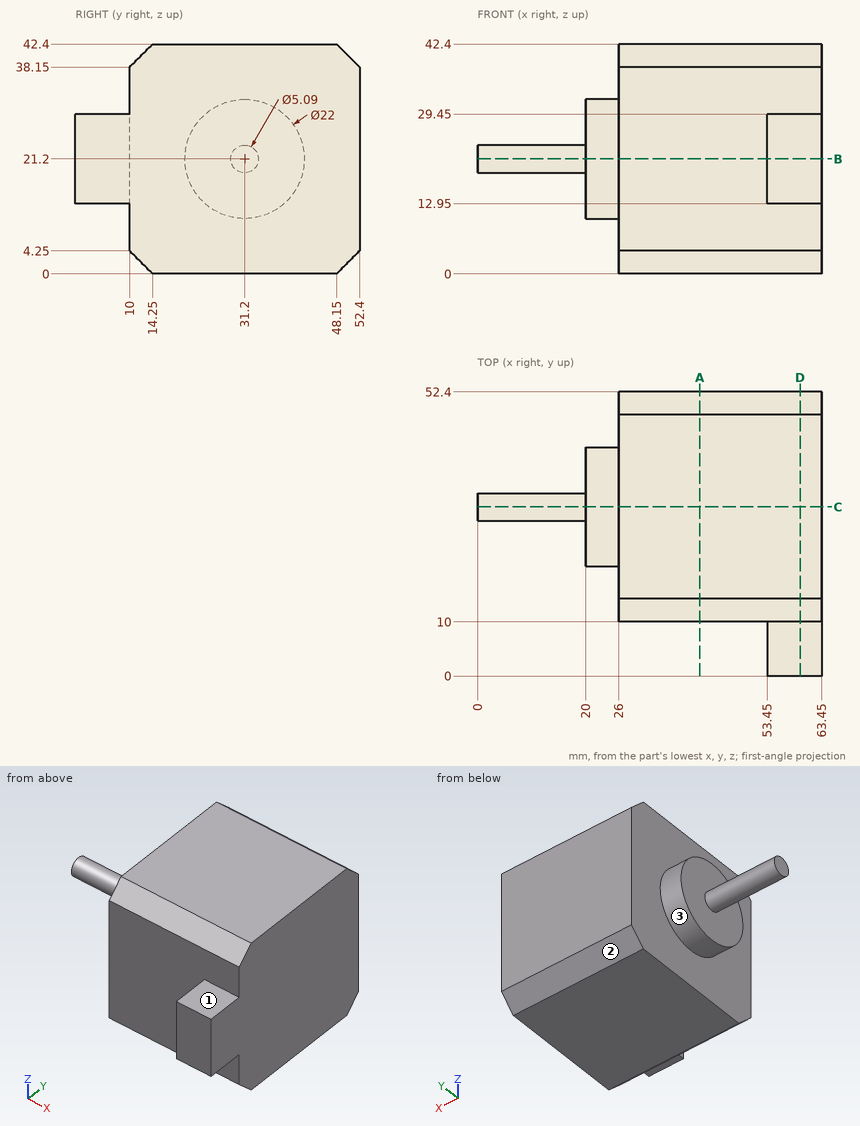
Here's the drawing with two shaded views (mm, measured from the low corner). I have some questions. A direction names the side the tool comes from. Coordinates: 2 decimals unless noted, no trailing zeros. Loops run counter-clockwise (first coordinate to the right, second up) from the corner with the lowest first, then second, coordinate; pieces in that order, holes last.
Item 1: I'm going to push flat-ended pins straight in: pin 1 (8 mm diameter, centred on y = 4, z = 18, fed in from -X); pin 2 (8 mm diameter, centred on x = 59.5, y = 6.5, fed in from -Z); pin 3 (12 mm diameter, centred on x = 12.5, z = 5, fed in from +Y); pin 4 (8 mm diameter, centred on x = 57, y = 3.5, fed in from +Z). Where does each tip first touch, or does it pass through?
Answers below:
pin 1: stops at x = 53.45
pin 2: stops at z = 3.75
pin 3: passes through
pin 4: stops at z = 29.45
Item 2: Please list where these lines run through material, in increasing order: L1, parallel to X at y = 7, z = 20.5; L2, parallel to X at y = 37.5, z = 32.5; L3, parallel to Y at x = 48, z = 24.
Answers below:
L1: x = 53.45 to 63.45
L2: x = 26 to 63.45
L3: y = 10 to 52.4
Item 3: Which directions (+Z, -Z, +X, -X, +Y, -Y) give clear straight access to the entire face, cutting with the end or side of a thin tool? Please do the marked faces 1, 2 and 3.
Answers below:
face 1: +Z, +X, -X, -Y
face 2: -Z, +X, -X, +Y
face 3: -X
Item 4: Suppose I cut it at A-A (x = 41). Please give me the cut outline in (y, z).
Answers below:
outline: (10, 4.25) - (14.25, 0) - (48.15, 0) - (52.4, 4.25) - (52.4, 38.15) - (48.15, 42.4) - (14.25, 42.4) - (10, 38.15) - close
Item 5: Suppose I cut it at C-C (y = 31.2). Please give me the cut outline in (x, z) (3 decimals), then the cut area to 3 significant figures.
Answers below:
outline: (0, 18.655) - (20, 18.655) - (20, 10.2) - (26, 10.2) - (26, 0) - (63.45, 0) - (63.45, 42.4) - (26, 42.4) - (26, 32.2) - (20, 32.2) - (20, 23.745) - (0, 23.745) - close
area: 1,820 mm2
Item 6: Suppose I cut it at D-D (x = 59.5). Please give me the cut outline in (y, z).
Answers below:
outline: (0, 12.95) - (10, 12.95) - (10, 4.25) - (14.25, 0) - (48.15, 0) - (52.4, 4.25) - (52.4, 38.15) - (48.15, 42.4) - (14.25, 42.4) - (10, 38.15) - (10, 29.45) - (0, 29.45) - close
Item 7: Suppose I cut it at B-B (z = 21.2). Please give me the cut outline in (x, y) (3 decimals), then the cut area to 3 significant figures.
Answers below:
outline: (0, 28.655) - (20, 28.655) - (20, 20.2) - (26, 20.2) - (26, 10) - (53.45, 10) - (53.45, 0) - (63.45, 0) - (63.45, 52.4) - (26, 52.4) - (26, 42.2) - (20, 42.2) - (20, 33.745) - (0, 33.745) - close
area: 1,920 mm2
